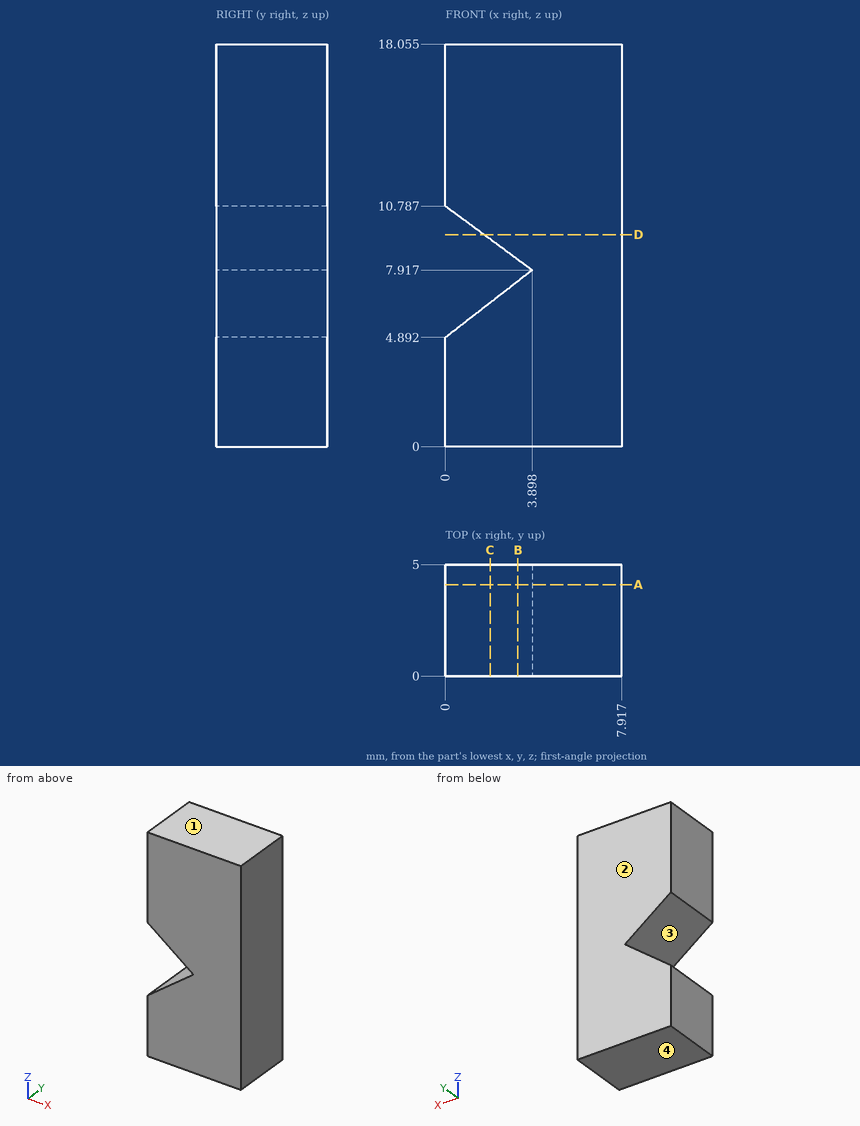
Source: three-view drawing plus pictorial views. Frame: mm from the lowest corner of the part. Give positions to 0.01 mm unless a question says otherwise; leave off trailing zeros. Order: outer loops, then holes, each group sorted by start corner. A loop starts at its lowest first (then second) coordinate and runs counter-clockwise, first axis right, second up. Notation, with made-up numbers: M 50.5,44 L 69.5,44 A11 ccw 69.5,57 Z; hole C -20,89 d8. An arc over 180 degrees is marked long. One line per question, with ' | ' between items.
1) Draft query along Z for the marked faces 1, 2, 3 and 4. Return one class per face: pulls with the +Z half, pulls with the -Z half, needs draft (parallel to the pull), parting line crosses it, or undercut.
Filled in:
face 1: pulls with the +Z half | face 2: needs draft | face 3: undercut | face 4: pulls with the -Z half
2) Contact query for a flat-ended pin moving along its axis: P1, Ø1.5, axis at y = 0.5, z = 10, coming from the -X side. Output: stop coordinate, or through.
Filled in:
P1: stops at x = 0.05
3) Section A-A on y = 4.1. Output: boundary loops of the cut face in (x, z) (1 decimal), and give its area (3 significant figures).
Filled in:
outline: M 0,0 L 7.9,0 L 7.9,18.1 L 0,18.1 L 0,10.8 L 3.9,7.9 L 0,4.9 Z | area: 131 mm2
4) Section B-B on x = 3.25. Output: boundary loops of the cut face in (y, z) (1 decimal).
Filled in:
outline: M 0,0 L 5,0 L 5,7.4 L 0,7.4 Z; M 0,8.4 L 5,8.4 L 5,18.1 L 0,18.1 Z
5) Ray query, L1, parallel to Z at x = 2.5, y = 0.75 (1 decimal); L2, parallel to X at y = 1.6, z = 8 (1 decimal); L3, parallel to Z at x = 3, y = 4.5 (1 decimal). Return the intervals inside material, ascending.
Filled in:
L1: z = 0 to 6.8, 8.9 to 18.1 | L2: x = 3.8 to 7.9 | L3: z = 0 to 7.2, 8.6 to 18.1
6) Section C-C on x = 2. Output: boundary loops of the cut face in (y, z) (1 decimal).
Filled in:
outline: M 0,0 L 5,0 L 5,6.4 L 0,6.4 Z; M 0,9.3 L 5,9.3 L 5,18.1 L 0,18.1 Z
7) Section D-D on z = 9.5. Output: boundary loops of the cut face in (x, y).
Filled in:
outline: M 1.75,0 L 7.92,0 L 7.92,5 L 1.75,5 Z
